Verification items for the finished model (mm, model axes). Coordinates: 2 decimals unless noted, no trailing zeros. Order: outer loops, then holes, each group sorted by start corner. A loop starts at its lowest first (then second) coordinate and runs counter-clockwise, first axis right, second up. Notation, with made-up numbers: (54.5, -37.75) -> (107.5, -37.75) arc R27 ccw to (107.5, -1.75) -> close; hole circle Ø9 at (86.25, 44.5). An arc over 180 degrees is marked (long way). Write item = value, one per line. Start each with the question number.
1. Go/stop test with flat-tipped pins: P1, Ø4, axis at x = -24.5, y = 13.5, coming from the -Z side; P2, Ø14.5, axis at x = -0.5, z = -9, coming from the -Y side; P3, Ø3, axis at x = -5.5, y = 12.5, coming from the -Z side. Record where each tip stops, or that it passes through.
2. Release check for a two-part mould opening along Z. For faces 1 (the cylindrical face through (-30.133, 11.117, -1.326)), 2 (the flat face through (0, 17.462, 0)), 3 (the cylindrical face through (-28.547, 11.09, -1.256)), 4 (the flat face through (-28.1, 9.525, 6.4)) record: +Z half, -Z half, draft (parallel to the pull), parting line (faces both ways), or undercut.
3. Cross-section at B-B on y = 16.5. Record the cut outline in (x, z).
4. Thickness scan on line 1 along Z through (x, y) = (0, 11.55) (1 decimal); line 2 along Y through (x, z) = (-1, -1.5). Record the ranges inside material, lowest first. Write a range as from..to.
from build123d import *

# Parameters (mm, degrees)
F2_SIZE = 0.8128


with BuildPart() as f1:
    # F0 (on Top) → F1 (revolve)
    with BuildSketch(Plane.XY):
        with BuildLine():
            Line((25.4, 19.05), (0, 19.05))
            Line((0, 19.05), (0, 17.4625))
            Line((0, 17.4625), (23.8125, 17.4625))
            ThreePointArc((23.8125, 17.4625), (27.180096, 16.067596), (28.575, 12.7))
            Line((28.575, 12.7), (28.575, 9.525))
            Line((28.575, 9.525), (30.1625, 9.525))
            Line((30.1625, 9.525), (30.1625, 11.8745))
            ThreePointArc((30.1625, 11.8745), (30.404283, 12.458217), (30.988, 12.7))
            Line((30.988, 12.7), (30.862477, 12.7))
            ThreePointArc((30.862477, 12.7), (31.488286, 12.987158), (31.678709, 13.648851))
            ThreePointArc((31.678709, 13.648851), (29.541093, 17.513923), (25.4, 19.05))
        make_face()
    revolve(axis=Axis((0, 18.25625, 0), (0, 1, 0)))

    # F2
    f2_edges = [f1.edges().sort_by_distance(p)[0] for p in [
        (-30.1625, 9.525, 0),
    ]]
    chamfer(f2_edges, length=F2_SIZE)


solid = f1.part
Worked out:
q1.P1 = -22.31
q1.P2 = 17.46
q1.P3 = -31.39
q2.face_1 = parting line
q2.face_2 = undercut
q2.face_3 = undercut
q2.face_4 = draft
q3.outline = circle Ø60.97 at (0, 0); hole circle Ø53.37 at (0, 0)
q4.line_1 = -30.2..-28.6, 28.6..30.2
q4.line_2 = 17.46..19.05
